Could you check a few things on this model? Use its own coordinates, in mm. A direction names the side the tool comes from. Round coordinates to 2 decimals unless told otherwise and drop trailing zeros. Loops run counter-clockwise (first coordinate to the right, second up) from the corner with the lowest first, then second, coordinate; pieces in that order, holes last.
from build123d import *

# Parameters (mm, degrees)
F0_R     = 3.175
F0_R_2   = 1.5875
F1_DEPTH = 3.048


with BuildPart() as f1:
    # F0 (on Front) → F1 (new body)
    with BuildSketch(Plane.XZ):
        with BuildLine():
            ThreePointArc((32.737635, 28.991633), (42.262635, 19.466633), (51.787635, 28.991633))
            ThreePointArc((51.787635, 28.991633), (42.262635, 38.516633), (32.737635, 28.991633))
        make_face()
        with Locations((42.262635, 28.991633)):
            Circle(F0_R, mode=Mode.SUBTRACT)
        with BuildLine():
            Line((57.491022, -18.011721), (51.787635, 28.991633))
            ThreePointArc((51.787635, 28.991633), (42.262635, 19.466633), (32.737635, 28.991633))
            Line((32.737635, 28.991633), (26.336892, -19.741037))
            ThreePointArc((26.336892, -19.741037), (41.196865, -5.957767), (57.491022, -18.011721))
        make_face()
        with Locations((36.633853, 14.716833)):
            Circle(F0_R_2, mode=Mode.SUBTRACT)
        with BuildLine():
            Line((57.951707, -21.808367), (57.491022, -18.011721))
            ThreePointArc((57.491022, -18.011721), (41.196865, -5.957767), (26.336892, -19.741037))
            ThreePointArc((26.336892, -19.741037), (26.238036, -22.881748), (26.759731, -25.980404))
            ThreePointArc((26.759731, -25.980404), (42.656766, -37.672766), (57.657464, -24.850672))
            Line((57.657464, -24.850672), (57.951707, -21.808367))
        make_face()
        with Locations((42.076707, -21.808367)):
            Circle(F0_R, mode=Mode.SUBTRACT)
        with BuildLine():
            ThreePointArc((57.951707, -21.808367), (57.836115, -19.89612), (57.491022, -18.011721))
            Line((57.491022, -18.011721), (57.951707, -21.808367))
        make_face()
        with BuildLine():
            ThreePointArc((57.657464, -24.850672), (57.877975, -23.336617), (57.951707, -21.808367))
            Line((57.951707, -21.808367), (57.657464, -24.850672))
        make_face()
        with BuildLine():
            ThreePointArc((57.657464, -24.850672), (42.656766, -37.672766), (26.759731, -25.980404))
            Line((26.759731, -25.980404), (32.760889, -85.192107))
            ThreePointArc((32.760889, -85.192107), (43.81357, -74.139426), (54.866251, -85.192107))
            ThreePointArc((54.866251, -85.192107), (51.916301, -92.709253), (44.64113, -96.213762))
            Line((44.64113, -96.213762), (88.748364, -95.124242))
            ThreePointArc((88.748364, -95.124242), (80.810864, -87.186742), (88.748364, -79.249242))
            Line((88.748364, -79.249242), (60.937904, -78.11713))
            ThreePointArc((60.937904, -78.11713), (55.267768, -75.396876), (53.347999, -69.408161))
            Line((53.347999, -69.408161), (57.657464, -24.850672))
        make_face()
        with BuildLine():
            ThreePointArc((54.866251, -85.192107), (43.81357, -74.139426), (32.760889, -85.192107))
            ThreePointArc((32.760889, -85.192107), (36.296423, -93.294838), (44.64113, -96.213762))
            ThreePointArc((44.64113, -96.213762), (51.916301, -92.709253), (54.866251, -85.192107))
        make_face()
        with Locations((43.81357, -85.192107)):
            Circle(F0_R, mode=Mode.SUBTRACT)
        with BuildLine():
            ThreePointArc((88.748364, -79.249242), (80.810864, -87.186742), (88.748364, -95.124242))
            ThreePointArc((88.748364, -95.124242), (94.361024, -92.799402), (96.685864, -87.186742))
            ThreePointArc((96.685864, -87.186742), (94.361024, -81.574082), (88.748364, -79.249242))
        make_face()
        with Locations((88.748364, -87.186742)):
            Circle(F0_R, mode=Mode.SUBTRACT)
    extrude(amount=F1_DEPTH)


solid = f1.part
Item 1: We'd pull the mould along X, two halves only. Please class faces 1 (the flat face through (45, -3.048, -43)), 2 (the flat face through (29.72, -1.5, -55.17)), 3 (the cylindrical face through (91.777, -1.503, -86.233)): released by +X, released by -X, zero draft, split by the parting line, or undercut.
Results list:
face 1: zero draft
face 2: released by -X
face 3: undercut
Item 2: If we section it at A-A, the plane x = 36.5: Please give me the cut outline in (y, z).
Results list:
outline: (-3.05, -93.48) - (0, -93.48) - (0, 13.13) - (-3.05, 13.13) - close; (-3.05, 16.3) - (0, 16.3) - (0, 36.58) - (-3.05, 36.58) - close
Item 3: If we section it at D-D, the plane x = 73: Please give me the cut outline in (y, z), then the cut area to 3 significant figures.
Results list:
outline: (-3.05, -95.51) - (0, -95.51) - (0, -78.61) - (-3.05, -78.61) - close
area: 51.5 mm2
Item 4: For faces 4 (the flat face through (55.473, -1.503, -47.441)), 5 (the flat face through (29.582, -1.503, 4.966)), which set-ups out of +Z, -Z, +X, -X, +Y, -Y let a thin tool reach every point of the face, with its end or its side?
Results list:
face 4: +X, +Y, -Y
face 5: +Z, -X, +Y, -Y
Item 5: If we section it at B-B, the plane y = -2.35: Count the separate pieces of the cut face and the enclosed holes in it, then the cut area to 3 significant figures.
Results list:
separate pieces: 1
enclosed holes: 5
area: 3,830 mm2
Item 6: If we section it at C-C, the plane z = -75.5: Please give me the cut outline in (x, y).
Results list:
outline: (31.78, -3.05) - (55.36, -3.05) - (55.36, 0) - (31.78, 0) - close
Item 7: If I drill on line 1 along Z through (x, y) = (42, -2.4); line 2 along Z through (x, y) = (46.5, -1.5); line 3 along Z through (x, y) = (91, -0.45), over which ranges is the centre line in solid material (lowest first)?
Results list:
line 1: z = -96.09 to -87.8, -82.59 to -24.98, -18.63 to 25.83, 32.16 to 38.51
line 2: z = -96.17 to -86.88, -83.5 to 37.52
line 3: z = -94.8 to -89.43, -84.95 to -79.58
Item 8: Will these pins go through, and if not, where does the flat tip stop? pin 1 (1.5 mm diameter, centred on y = -0.5, z = 18, fed in from -X); pin 2 (5.5 mm diameter, centred on x = 88.75, z = -87.19, fed in from +Y).
Results list:
pin 1: stops at x = 31.2
pin 2: passes through
